from build123d import *

# Parameters (mm, degrees)
F0_R          = 38.1
F1_DEPTH      = 38.1
F1_DEPTH_BACK = 38.1
F2_R          = 38.09999
F3_R          = 38.09999
F4_R          = 3.175
F5_DEPTH      = 152.4
F6_R          = 15
F7_DEPTH      = 15
F7_DEPTH_BACK = 15
F8_R          = 15


# Not quite as in the source:
# - a fillet or chamfer that OpenCascade refuses, or shapes differently, is made with other operations: its cross-section is extruded or revolved along the edge and cut away or added
# - a fillet or chamfer is up to 0.001 mm smaller than in the source, because OpenCascade refuses the exact size
# - the program builds the solid bodies; features that only make, move or delete a surface that nothing else refers to are left out


with BuildPart() as f1:
    # F0 (on Top) → F1 (new body, two sides)
    with BuildSketch(Plane.XY) as f1_sk:
        Circle(F0_R)
    extrude(amount=F1_DEPTH)
    extrude(f1_sk.sketch, amount=-F1_DEPTH_BACK)

    # F2 (radius 38.1 in the source; OpenCascade refuses exactly that, so slightly less here)
    f2_edges = [f1.edges().sort_by_distance(p)[0] for p in [
        (-38.1, 0, 38.1),
    ]]
    fillet(f2_edges, radius=F2_R)

    # F3 (radius 38.1 in the source; OpenCascade refuses exactly that, so slightly less here)
    f3_edges = [f1.edges().sort_by_distance(p)[0] for p in [
        (-38.1, 0, -38.1),
    ]]
    fillet(f3_edges, radius=F3_R)

    # F4 (on Top) → F5 (join)
    with BuildSketch(Plane.XY):
        Circle(F4_R)
    extrude(amount=F5_DEPTH)

    # F6 (on face) → F7 (join, two sides)
    with BuildSketch(Plane.XY.offset(152.4)) as f7_sk:
        Circle(F6_R)
    extrude(amount=F7_DEPTH)
    extrude(f7_sk.sketch, amount=-F7_DEPTH_BACK)

    # F8
    f8_edges = [f1.edges().sort_by_distance(p)[0] for p in [
        (-15, 0, 167.4),
    ]]
    fillet(f8_edges, radius=F8_R)

    # F9: fillet of radius 14.999 on 1 edges, made by hand

    # F9_s1 → F9_t2 (revolve, cut)
    with BuildSketch(Plane.XZ):
        with BuildLine():
            ThreePointArc((15, 152.0593221194), (11.6752628675, 142.6422319372), (3.175, 137.4))
            Line((3.175, 137.4), (15, 137.4))
            Line((15, 137.4), (15, 152.0593221194))
        make_face()
    revolve(axis=Axis((0, 0, 137.4), (0, 0, 1)), mode=Mode.SUBTRACT)


solid = f1.part
Geometry check sheet. Reference: the model listing, model coordinates, mm. A direction names the side the tool comes from. Round coordinates to 2 decimals unless told otherwise and drop trailing zeros. Loops run counter-clockwise (first coordinate to the right, second up) from the corner with the lowest first, then second, coordinate; pieces in that order, holes last. Notation, with made-up numbers: (18, -0.75) -> (54, -0.75) arc R26 cw to (54, 36.25) -> close; hole circle Ø10 at (15.5, 44.5). An arc over 180 degrees is marked (long way). Answer as a JSON object with one key per item and string values. Group by question number.
Item 1: Set-up check for faces 1 (the face through (-0.69, -3.1, 86.99)), 2 (the face through (-14.985, 0.66, 152.232)): record each of +Z, -Z, +X, -X, +Y, -Y from which the full face is reachable in a straight line by a thin tool's end or side.
Item 2: Depth check by flat-ended pin: pin 1 Ø3 at (x, y) = (30.5, -15.5) entering from +Z; pin 2 Ø3 at (x, y) = (6.5, 19.5) entering from -Z; pin 3 Ø10 at (x, y) = (-3, -3) entering from +Z; pin 4 Ø1 at (x, y) = (6, -3) entering from +Z (3 decimals). Enter the tip coordinate at first touch or a pass-through.
Item 3: Thickness scan on line 1 along X through (y, z) = (2, 49). Record the ranges inside material, lowest first.
Item 4: Cross-section at A-A, the plane z = 123.5. Record the cut outline in (x, y) (3 decimals), plus the area to 3 significant figures.
Determined:
{
 "1": {"face 1": "none", "face 2": "+Z"},
 "2": {"pin 1": "stops at z = 19.53", "pin 2": "stops at z = -32.99", "pin 3": "stops at z = 167.4", "pin 4": "stops at z = 166.055"},
 "3": {"line 1": "x = -2.47 to 2.47"},
 "4": {"outline": "circle Ø6.35 at (0, 0)", "area": "31.7 mm²"}
}
